Drawing for the job (mm, zero at the part's lowest x, y, z). Give positions to 0.01 mm unless a question says otherwise; leave off trailing zeros. Order: outer loops, then holes, each group sorted by start corner. A loop starts at its lowest first (then second) coordinate and runs counter-clockwise, first axis right, second up. Notation, with made-up numbers: (53, 63) - (103, 63) arc R19 ccw to (103, 78) - close; hole circle Ø1 at (17.5, 35). An arc over 180 degrees is marked (long way). One line per item, written item: value.
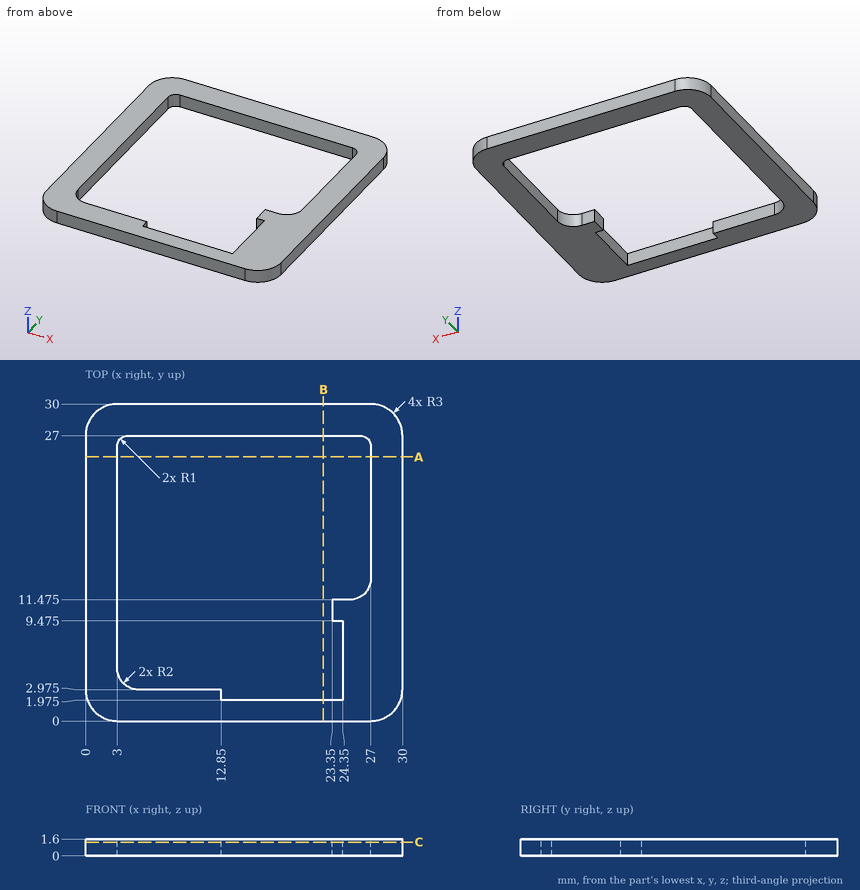
1) Pin check, flat tips, straight feed: pin 1 (6 mm diameter, centred on x = 11, y = 7, fed in from +Z); pin 2 (0.5 mm diameter, centred on y = 2.5, z = 0.5, fed in from +X). Stop position of each tip, or through.
Outcome:
pin 1: passes through
pin 2: stops at x = 29.99
2) Cut at A-A, the plane y = 25. Give the cut face in (x, z).
Outcome:
outline: (0, 0) - (3, 0) - (3, 1.6) - (0, 1.6) - close; (27, 0) - (30, 0) - (30, 1.6) - (27, 1.6) - close
3) Drill centre lines: line 1 along Y through (x, z) = (8.75, 1.1) (3 decimals); line 2 along Y through (x, z) = (15.75, 0.1) (3 decimals); line 3 along X through (y, z) = (21, 1.25). Where is each one in solid material? Low to high. Write a range as from..to.
Outcome:
line 1: y = 0..2.975, 27..30
line 2: y = 0..1.975, 27..30
line 3: x = 0..3, 27..30
4) Cut at C-C, the plane z = 1.3. Give the cut face in (x, y) (3 decimals).
Outcome:
outline: (0, 3) arc R3 ccw to (3, 0) - (27, 0) arc R3 ccw to (30, 3) - (30, 27) arc R3 ccw to (27, 30) - (3, 30) arc R3 ccw to (0, 27) - close; hole (3, 4.975) arc R2 ccw to (5, 2.975) - (12.85, 2.975) - (12.85, 1.975) - (24.35, 1.975) - (24.35, 9.475) - (23.35, 9.475) - (23.35, 11.475) - (25, 11.475) arc R2 ccw to (27, 13.475) - (27, 26) arc R1 ccw to (26, 27) - (4, 27) arc R1 ccw to (3, 26) - close
5) Cut at B-B, the plane x = 22.5. Give the cut face in (y, z) (3 decimals).
Outcome:
outline: (0, 0) - (1.975, 0) - (1.975, 1.6) - (0, 1.6) - close; (27, 0) - (30, 0) - (30, 1.6) - (27, 1.6) - close
